```python
from build123d import *

# Parameters (mm, degrees)
ESQUISSE2_W             = 50
ESQUISSE2_H             = 17
ESQUISSE3_W             = 40
ESQUISSE3_H             = 40
ENL_V_MAT_EXTRU_1_DEPTH = 25
ENL_V_START             = -25
ESQUISSE3_3_W           = 40
ESQUISSE3_3_H           = 40
ENL_V_MAT_EXTRU_2_DEPTH = 25
ENL_V_MAT_EXTRU_2_DRAFT = -20


with BuildPart() as part:
    # Esquisse1 → Révolution1 (revolve)
    with BuildSketch(Plane.XY, mode=Mode.PRIVATE) as r_volution1_sk:
        Polygon((650, 0), (650, 17.5), (156, 17.5), (156, 100), (138, 100), (138, 17.5), (58.6, 17.5), (41, 35), (0, 35), (0, 0), align=None)
    revolve(r_volution1_sk.sketch.rotate(Axis((0, 0, 0), (1, 0, 0)), 90), axis=Axis((0, 0, 0), (1, 0, 0)))

    # Esquisse2 → Révolution2 (revolve)
    with BuildSketch(Plane.XY, mode=Mode.PRIVATE) as r_volution2_sk:
        with Locations((181, 72.5)):
            Rectangle(ESQUISSE2_W, ESQUISSE2_H)
    revolve(r_volution2_sk.sketch.rotate(Axis((156, 64, 0), (1, 0, 0)), 90), axis=Axis((156, 64, 0), (1, 0, 0)))

    # Esquisse3 → Enlèv. mat.-Extru.1 (cut)
    with BuildSketch(Plane.ZY):
        Rectangle(ESQUISSE3_W, ESQUISSE3_H)
    extrude(amount=-ENL_V_MAT_EXTRU_1_DEPTH, mode=Mode.SUBTRACT)


with BuildPart() as enl_v_mat_extru_2_tool:
    # Esquisse3<3> → Enlèv. mat.-Extru.2 (with draft: the straight prism first)
    with BuildSketch(Plane.ZY.offset(ENL_V_START)):
        Rectangle(ESQUISSE3_3_W, ESQUISSE3_3_H)
    extrude(amount=-ENL_V_MAT_EXTRU_2_DEPTH)
    # Enlèv. mat.-Extru.2: the draft: its side faces are tilted about the plane it starts from
    enl_v_mat_extru_2_sides = [enl_v_mat_extru_2_tool.faces().sort_by_distance(p)[0] for p in [
        (37.5, 0, -20),
        (37.5, -20, 0),
        (37.5, 0, 20),
        (37.5, 20, 0),
    ]]
    draft(enl_v_mat_extru_2_sides, Plane.ZY.offset(ENL_V_START), ENL_V_MAT_EXTRU_2_DRAFT)


with BuildPart() as part_1:
    add(part.part)

    # Enlèv. mat.-Extru.2: cut by enl_v_mat_extru_2_tool
    add(enl_v_mat_extru_2_tool.part, mode=Mode.SUBTRACT)


solid = part_1.part
```
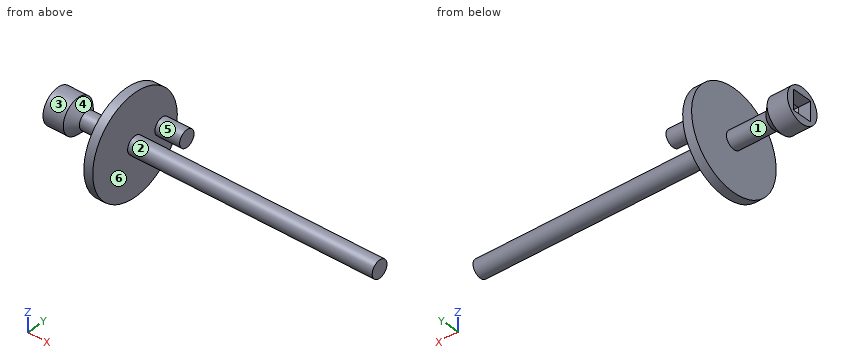
Can you work these out from the model? Positions are in its coordinate system, mm. Face numbers are marked on the shaded views. A direction names the side the tool comes from. Give positions to 0.01 mm unless a question says otherwise; leave off trailing zeros. Write each loop counter-clockwise with the first axis right and the second up, starting at its lowest first coordinate (ties: lowest second). Pieces come first, ordered by that corner, then holes. Notation, with made-up numbers: (51.25, 30) - (84.25, 30) arc R27 cw to (84.25, 65) - close; hole circle Ø8 at (15, 42.5). An arc over 180 degrees is marked (long way). Write item = value, one per line. Start each with the question number.
1. Imagine slicing it at C-C (x = 427). Please give me the cut outline in (y, z), and give its area (3 significant figures).
2. Thinking about a two-plate mould opening in X: for the marked faces 4, 5 and 6, which applies, released by +X, released by -X, zero draft, split by the parting line, or undercut?
3. Imagine slicing it at D-D (y = 64). Please give me the cut outline in (x, z).
4. For pin 1 (12.5 mm diameter, centred on x = 13.5, y = -6.5, fed in from +Z); pin 2 (2 mm diameter, centred on y = -71, z = -54, fed in from -X); pin 3 (1 mm diameter, centred on y = -32, z = -56.5, fed in from +X), each with a flat end and sliding along its axis, tell me the tip position at first contact or that it passes through.
5. On a 3-axis mill with a long thin cutter (end or side, diameter ignored), from which of +Z, -Z, +X, -X, +Y, -Y can I reach the whole of each face in a straight line? I mean the marked faces 1, 2 and 3. Say none if no direction works.
6. Imagine slicing it at B-B (z = 0). Please give me the cut outline in (x, y), and give its area (3 significant figures).
7. Please list where these lines run through material, in increasing order: line 1 (X direction, y = -57.5, z = 14.5); line 2 (Z direction, x = 187.5, y = -1.5); line 3 (X direction, y = 5.5, z = -10.5).
8. Imagine slicing it at A-A (y = 0). Please give me the cut outline in (x, z).
Worked answers:
q1.outline = circle Ø35 at (0, 0)
q1.area = 962 mm2
q2.face_4 = undercut
q2.face_5 = zero draft
q2.face_6 = released by +X
q3.outline = (138, -76.84) - (156, -76.84) - (156, -17) - (206, -17) - (206, 17) - (156, 17) - (156, 76.84) - (138, 76.84) - close
q4.pin_1 = 35
q4.pin_2 = 138
q4.pin_3 = 156
q5.face_1 = none
q5.face_2 = +X
q5.face_3 = -X
q6.outline = (0, -35) - (41, -35) - (58.6, -17.5) - (138, -17.5) - (138, -100) - (156, -100) - (156, -17.5) - (650, -17.5) - (650, 17.5) - (156, 17.5) - (156, 47) - (206, 47) - (206, 81) - (156, 81) - (156, 100) - (138, 100) - (138, 17.5) - (58.6, 17.5) - (41, 35) - (0, 35) - (0, 20) - (25, 20) - (50, 10.9) - (50, -10.9) - (25, -20) - (0, -20) - close
q6.area = 27,400 mm2
q7.line_1 = 138 to 156
q7.line_2 = -17.44 to 17.44
q7.line_3 = 50 to 650
q8.outline = (0, -35) - (41, -35) - (58.6, -17.5) - (138, -17.5) - (138, -100) - (156, -100) - (156, -17.5) - (650, -17.5) - (650, 17.5) - (156, 17.5) - (156, 100) - (138, 100) - (138, 17.5) - (58.6, 17.5) - (41, 35) - (0, 35) - (0, 20) - (25, 20) - (50, 10.9) - (50, -10.9) - (25, -20) - (0, -20) - close
